from build123d import *

# Parameters (mm, degrees)
F0_W     = 500
F0_H     = 500
F0_R     = 6
F0_W_2   = 400
F0_H_2   = 400
F1_DEPTH = 30
F6_F1_R  = 5
F6_F2_R  = 5
F6_F3_R  = 5


with BuildPart() as f1:
    # F0 (on Top) → F1 (new body)
    with BuildSketch(Plane.XY):
        Rectangle(F0_W, F0_H)
        with Locations((-225, -225)):
            Circle(F0_R, mode=Mode.SUBTRACT)
        with Locations((225, -225)):
            Circle(F0_R, mode=Mode.SUBTRACT)
        with Locations((-225, 225)):
            Circle(F0_R, mode=Mode.SUBTRACT)
        Rectangle(F0_W_2, F0_H_2, mode=Mode.SUBTRACT)
        with Locations((225, 225)):
            Circle(F0_R, mode=Mode.SUBTRACT)
    extrude(amount=F1_DEPTH)

    # F6: fillet of radius 5 on 22 edges, made by hand

    # F6_f1
    f6_f1_edges = [f1.edges().sort_by_distance(p)[0] for p in [
        (-200, -200, 15),
        (-200, 200, 15),
        (200, 200, 15),
        (200, -200, 15),
    ]]
    fillet(f6_f1_edges, radius=F6_F1_R)

    # F6_f2
    f6_f2_edges = [f1.edges().sort_by_distance(p)[0] for p in [
        (250, -250, 15),
        (250, 250, 15),
        (250, 0, 0),
        (250, 0, 30),
        (-250, 250, 15),
        (0, 250, 0),
        (0, 250, 30),
        (-250, 0, 30),
        (-250, -250, 15),
        (-250, 0, 0),
        (0, -250, 0),
        (0, -250, 30),
    ]]
    fillet(f6_f2_edges, radius=F6_F2_R)

    # F6_f3
    f6_f3_edges = [f1.edges().sort_by_distance(p)[0] for p in [
        (-200, 0, 0),
        (-200, 0, 30),
        (0, 200, 0),
        (0, 200, 30),
        (0, -200, 0),
        (0, -200, 30),
        (198.5355339059, -198.5355339059, 30),
        (-198.5355339059, -198.5355339059, 30),
        (198.5355339059, -198.5355339059, 0),
        (-198.5355339059, -198.5355339059, 0),
        (-198.5355339059, 198.5355339059, 30),
        (198.5355339059, 198.5355339059, 30),
        (-198.5355339059, 198.5355339059, 0),
        (198.5355339059, 198.5355339059, 0),
    ]]
    fillet(f6_f3_edges, radius=F6_F3_R)


solid = f1.part
For this review, take the finished solid that the model builds, in its own axes (mm). A direction names the side the tool comes from. Give positions to 0.01 mm unless a question says otherwise; leave off trailing zeros. Loops run counter-clockwise (first coordinate to the right, second up) from the corner with the lowest first, then second, coordinate; pieces in that order, holes last.
Item 1: Insertion check: pin 1 (6 mm diameter, centred on y = -122.5, z = 3, fed in from -X); pin 2 (7 mm diameter, centred on x = 225, y = 225, fed in from -Z). Each pin has a flat end and moves straight along its axis. Give the tip position at first contact, or say it passes through.
Item 2: Take a section at C-C, the plane x = -16. State the section outline as (y, z) points.
Item 3: For line 1 along Y through (x, z) = (-225, 21); line 2 along X through (y, z) = (141.5, 11.25), list the stretches that pass through material, from the lowest coordinate up.
Item 4: Tool access review of faces 1 (the flat face through (-250, -3, 15)), 2 (the flat face through (-200, -3, 15)): name each direction out of +Z, -Z, +X, -X, +Y, -Y from which nothing blocks a thin tool from reaching the whole face with its end or side.
Item 5: Take a section at A-A, the plane z = 20.5. State the section outline as (x, y) points, and give its area (3 significant figures).
Item 6: Take a section at B-B, the plane y = -225. State the section outline as (x, z) points.
Calculated:
1. pin 1: stops at x = -250
1. pin 2: passes through
2. outline: (-250, 5) arc R5 ccw to (-245, 0) - (-205, 0) arc R5 ccw to (-200, 5) - (-200, 25) arc R5 ccw to (-205, 30) - (-245, 30) arc R5 ccw to (-250, 25) - close; (200, 5) arc R5 ccw to (205, 0) - (245, 0) arc R5 ccw to (250, 5) - (250, 25) arc R5 ccw to (245, 30) - (205, 30) arc R5 ccw to (200, 25) - close
3. line 1: y = -250 to -231, -219 to 219, 231 to 250
3. line 2: x = -250 to -200, 200 to 250
4. face 1: +Z, -Z, -X, +Y, -Y
4. face 2: +Z, -Z
5. outline: (-250, -245) arc R5 ccw to (-245, -250) - (245, -250) arc R5 ccw to (250, -245) - (250, 245) arc R5 ccw to (245, 250) - (-245, 250) arc R5 ccw to (-250, 245) - close; hole circle Ø12 at (-225, -225); hole circle Ø12 at (-225, 225); hole (-200, -195) arc R5 ccw to (-195, -200) - (195, -200) arc R5 ccw to (200, -195) - (200, 195) arc R5 ccw to (195, 200) - (-195, 200) arc R5 ccw to (-200, 195) - close; hole circle Ø12 at (225, -225); hole circle Ø12 at (225, 225)
5. area: 89,500 mm2
6. outline: (-250, 5) arc R5 ccw to (-245, 0) - (-231, 0) - (-231, 30) - (-245, 30) arc R5 ccw to (-250, 25) - close; (-219, 0) - (219, 0) - (219, 30) - (-219, 30) - close; (231, 0) - (245, 0) arc R5 ccw to (250, 5) - (250, 25) arc R5 ccw to (245, 30) - (231, 30) - close
